Answer from the drawing. Dimensions are ordinates in mm from the lowest x, y and z of the part. Round coordinates to 2 decimals unless told otherwise and drop trailing zeros. Loops run counter-clockwise (first coordinate to the right, second up) from the corner with the lowest first, then second, coordinate; pieces in that order, holes last. Notation, with made-up numbers: (-9.5, -25) - (-5.5, -25) arc R21 cw to (-5.5, -3) - close; hole circle Ø9 at (51, -13). An arc over 180 degrees is marked (long way). Return JSON: item names as keys, results as strings.
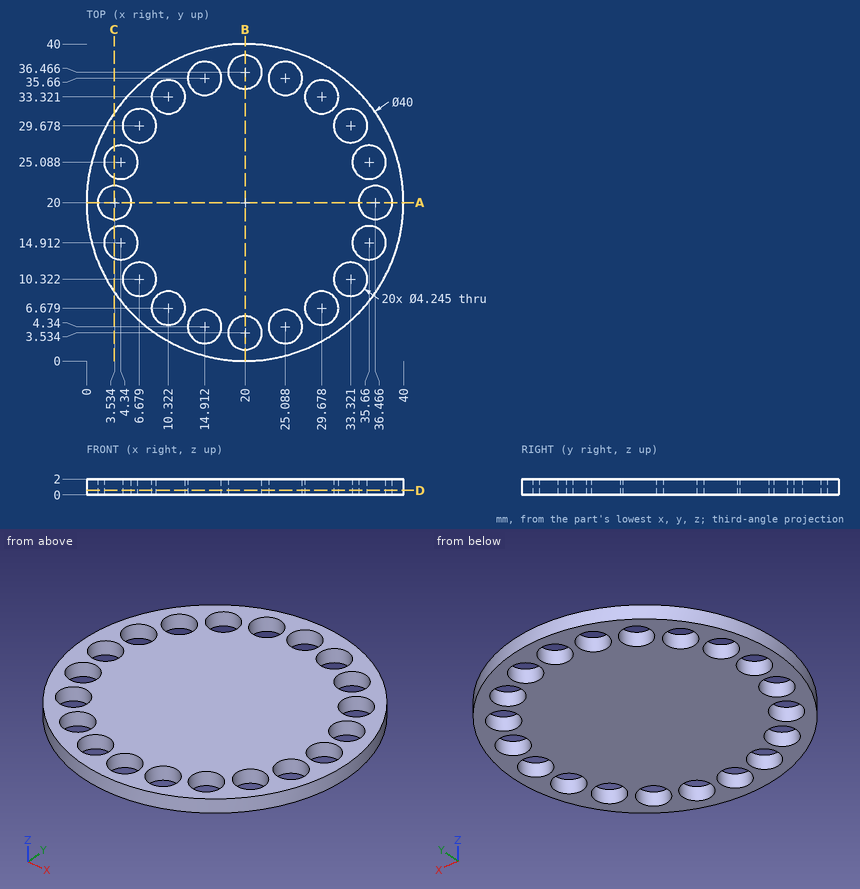
1) Find the intervals of material crossed by L1, parallel to Y at x = 20, z = 1; L2, parallel to Y at x = 11.5, z = 0.55 (1 decimal); L3, parallel to X at y = 30.5, z = 0.9 (1 decimal), in increasing order.
Verdict:
{"L1": "y = 0 to 1.41, 5.66 to 34.34, 38.59 to 40", "L2": "y = 1.9 to 4.9, 8.4 to 31.6, 35.1 to 38.1", "L3": "x = 3 to 4.7, 8.6 to 31.4, 35.3 to 37"}
2) Section A-A (y = 20) is taken. Give the vertices of the cut face in (x, z).
Verdict:
{"outline": "(0, 0) - (1.41, 0) - (1.41, 2) - (0, 2) - close; (5.66, 0) - (34.34, 0) - (34.34, 2) - (5.66, 2) - close; (38.59, 0) - (40, 0) - (40, 2) - (38.59, 2) - close"}
3) Section D-D (z = 0.55) is taken. Count the separate pieces of the cut face and the enclosed holes in it.
Verdict:
{"separate pieces": "1", "enclosed holes": "20"}
4) Section C-C (x = 3.5) is taken. Give the vertices of the cut face in (y, z).
Verdict:
{"outline": "(8.7, 0) - (12.96, 0) - (12.96, 2) - (8.7, 2) - close; (16.86, 0) - (17.88, 0) - (17.88, 2) - (16.86, 2) - close; (22.12, 0) - (23.14, 0) - (23.14, 2) - (22.12, 2) - close; (27.04, 0) - (31.3, 0) - (31.3, 2) - (27.04, 2) - close"}
5) A flat-ended cylindrical pin translates along its axis: pin 1 (1 mm diameter, centred on x = 27, z = 0.5, fed in from +Y) (1 decimal). Find the tip coordinate at first contact, or state that the pin passes through.
Verdict:
{"pin 1": "stops at y = 38.9"}
